The listing builds one solid part. Answer for the finished solid, in the listing's coordinates (mm). A direction names the side the tool comes from. Give positions to 0.01 mm unless a question says otherwise; leave off trailing zeros. Write each loop counter-clockwise with the first axis right and the second up, starting at its lowest first coordinate (ties: lowest second). Pieces come first, ordered by that corner, then holes. Notation, with made-up numbers: (47.25, 5.5) - (86.25, 5.5) arc R17 cw to (86.25, 29.5) - close; hole circle Ø3 at (22.25, 49.5). An arc over 180 degrees is marked (long way). Write each question's results on one line, items separated by ' | '. Start each with the question number.
Q1. Flat-ended cylindrical pins translate along their axes: pin 1 Ø5 at (x, y) = (1564, 48.5) entering from +Z; pin 2 Ø1.5 at (x, y) = (1458.5, -203.5) entering from -Z; pin 3 Ø3 at (y, z) = (-48, 861.5) entering from -X. Find the tip coordinate at first contact, or state that the pin passes through.
Q2. Section D-D (x = 914.4) is taken. Determine the outline of the cut face in (y, z), plus the area to 3 significant figures.
Q3. For a pull along Z with two mould halves and no side action, classify faces 1 (the face through (1176.867, -3, 431)), 2 (the face through (906, 50.8, 952)), 3 (the face through (1508.304, -241.122, 259.722)) as pulls with the +Z half, pulls with the -Z half, needs draft (parallel to the pull), parting line crosses it, or undercut.
Q4. For faces 4 (the face through (1376, -1, 609.6)), 5 (the face through (911, -50.8, 632)), 6 (the face through (76.2, -3, 431)), 7 (the face through (336.19, -241.12, 272.89)), determine the directions among +Z, -Z, +X, -X, +Y, -Y from which every point of the face is accessible in a straight line to the end or side of a thin tool.
Q5. Section A-A (z = 453.5) is taken. Determine the outline of the cut face in (x, y).
Q6. Section C-C (y = 90) is taken. Determine the outline of the cut face in (x, z), plus the area to 3 significant figures.
Q7. Section B-B (x = 1324) is taken. Determine the outline of the cut face in (y, z), plus the area to 3 significant figures.
Q8. Find the intervals of material crossed by probe 1 along Z at (x, y) = (1495.5, 17.5); probe 2 along Z at (x, y) = (1694, -99); probe 3 along Z at (x, y) = (957, -85), in increasing order.
```python
from build123d import *

# Parameters (mm, degrees)
F0_W      = 76.2
F0_H      = 127
F0_W_2    = 50.8
F0_H_2    = 101.6
F1_DEPTH  = 228.6
F2_W      = 304.8
F2_H      = 127
F3_DEPTH  = 1828.801
F0_W_3    = 584.2
F0_H_3    = 50.8
F4_DEPTH  = 50.8
F5_W      = 584.2
F5_H      = 228.6
F6_DEPTH  = 12.7
F7_R      = 19.05
F8_DEPTH  = 25.4
F9_W      = 1239.3679447479
F9_H      = 644.6519196678
F10_DEPTH = 6.35


with BuildPart() as f1:
    # F0 (on Front) → F1 (new body, symmetric)
    with BuildSketch(Plane.XZ):
        Polygon((0, 558.8), (0, 127), (76.2, 127), (1752.6, 127), (1828.8, 127), (1828.8, 558.8), (1206.5, 558.8), (622.3, 558.8), align=None)
        Polygon((76.2, 381), (76.2, 482.6), (601.1333333333, 482.6), (651.9333333333, 482.6), (1176.8666666667, 482.6), (1227.6666666667, 482.6), (1752.6, 482.6), (1752.6, 381), (1227.6666666667, 381), (1176.8666666667, 381), (651.9333333333, 381), (601.1333333333, 381), align=None, mode=Mode.SUBTRACT)
        with Locations((38.1, 63.5)):
            Rectangle(F0_W, F0_H)
        with Locations((1790.7, 63.5)):
            Rectangle(F0_W, F0_H)
        with Locations((626.5333333333, 431.8)):
            Rectangle(F0_W_2, F0_H_2)
        with Locations((1202.2666666667, 431.8)):
            Rectangle(F0_W_2, F0_H_2)
    extrude(amount=F1_DEPTH, both=True)

    # F2 (on face) → F3 (cut, through all)
    with BuildSketch(Plane.YZ.offset(1828.8)):
        with Locations((0, 63.5)):
            Rectangle(F2_W, F2_H)
    extrude(amount=-F3_DEPTH, mode=Mode.SUBTRACT)

    # F0 (on Front) → F4 (join, symmetric)
    with BuildSketch(Plane.XZ):
        Polygon((279.4, 609.6), (622.3, 609.6), (1206.5, 609.6), (1549.4, 609.6), (1549.4, 1333.5), (279.4, 1333.5), align=None)
        with Locations((914.4, 584.2)):
            Rectangle(F0_W_3, F0_H_3)
    extrude(amount=F4_DEPTH, both=True)

    # F5 (on face) → F6 (join)
    with BuildSketch(Plane.XY.offset(558.8)):
        with Locations((915.0145053864, 0)):
            Rectangle(F5_W, F5_H)
    extrude(amount=F6_DEPTH)

    # F7 (on face) → F8 (join)
    with BuildSketch(Plane.XZ.offset(228.6)):
        with Locations((338.6666666667, 254)):
            Circle(F7_R)
        with Locations((914.4, 254)):
            Circle(F7_R)
        with Locations((1490.1333333333, 254)):
            Circle(F7_R)
    extrude(amount=F8_DEPTH)

    # F9 (on face) → F10 (cut)
    with BuildSketch(Plane.XZ.offset(50.8)):
        with Locations((914.7072526932, 975.6220156918)):
            Rectangle(F9_W, F9_H)
    extrude(amount=-F10_DEPTH, mode=Mode.SUBTRACT)


solid = f1.part
```
Answers below:
1) pin 1: stops at z = 558.8 | pin 2: stops at z = 127 | pin 3: stops at x = 279.4
2) outline: (-254, 234.95) - (-228.6, 234.95) - (-228.6, 127) - (228.6, 127) - (228.6, 381) - (-228.6, 381) - (-228.6, 273.05) - (-254, 273.05) - close; (-228.6, 482.6) - (228.6, 482.6) - (228.6, 558.8) - (114.3, 558.8) - (114.3, 571.5) - (50.8, 571.5) - (50.8, 1333.5) - (-50.8, 1333.5) - (-50.8, 1297.95) - (-44.45, 1297.95) - (-44.45, 653.3) - (-50.8, 653.3) - (-50.8, 571.5) - (-114.3, 571.5) - (-114.3, 558.8) - (-228.6, 558.8) - close | area: 228,000 mm2
3) face 1: undercut | face 2: needs draft | face 3: parting line crosses it
4) face 4: +X, +Y, -Y | face 5: +Z, +X, -X, -Y | face 6: +Y, -Y | face 7: -Y
5) outline: (0, -228.6) - (76.2, -228.6) - (76.2, 228.6) - (0, 228.6) - close; (601.13, -228.6) - (651.93, -228.6) - (651.93, 228.6) - (601.13, 228.6) - close; (1176.87, -228.6) - (1227.67, -228.6) - (1227.67, 228.6) - (1176.87, 228.6) - close; (1752.6, -228.6) - (1828.8, -228.6) - (1828.8, 228.6) - (1752.6, 228.6) - close
6) outline: (0, 127) - (1828.8, 127) - (1828.8, 558.8) - (1207.11, 558.8) - (1207.11, 571.5) - (622.91, 571.5) - (622.91, 558.8) - (0, 558.8) - close; hole (76.2, 381) - (601.13, 381) - (601.13, 482.6) - (76.2, 482.6) - close; hole (651.93, 381) - (1176.87, 381) - (1176.87, 482.6) - (651.93, 482.6) - close; hole (1227.67, 381) - (1752.6, 381) - (1752.6, 482.6) - (1227.67, 482.6) - close | area: 637,000 mm2
7) outline: (-228.6, 127) - (228.6, 127) - (228.6, 381) - (-228.6, 381) - close; (-228.6, 482.6) - (228.6, 482.6) - (228.6, 558.8) - (-228.6, 558.8) - close; (-50.8, 609.6) - (50.8, 609.6) - (50.8, 1333.5) - (-50.8, 1333.5) - (-50.8, 1297.95) - (-44.45, 1297.95) - (-44.45, 653.3) - (-50.8, 653.3) - close | area: 220,000 mm2
8) probe 1: z = 127 to 381, 482.6 to 558.8, 609.6 to 1333.5 | probe 2: z = 127 to 381, 482.6 to 558.8 | probe 3: z = 127 to 381, 482.6 to 571.5
